Source: three-view drawing plus pictorial views. Frame: mm from the lowest corner of the part. A direction names the side the tool comes from. Give positions to 0.01 mm unless a question says otherwise; leave off trailing zeros. Write each loop counter-clockwise with the first axis right and the second up, starting at its lowest first coordinate (ties: lowest second). Pieces come first, ordered by that corner, then holes. Notation, with made-up numbers: (8.5, 50.5) -> (50.5, 50.5) arc R32 ccw to (50.5, 82.5) -> close; hole circle Ø5 at (46.5, 26). An arc over 180 degrees is marked (long way). Use a Markdown table: item, result. Add a question column.
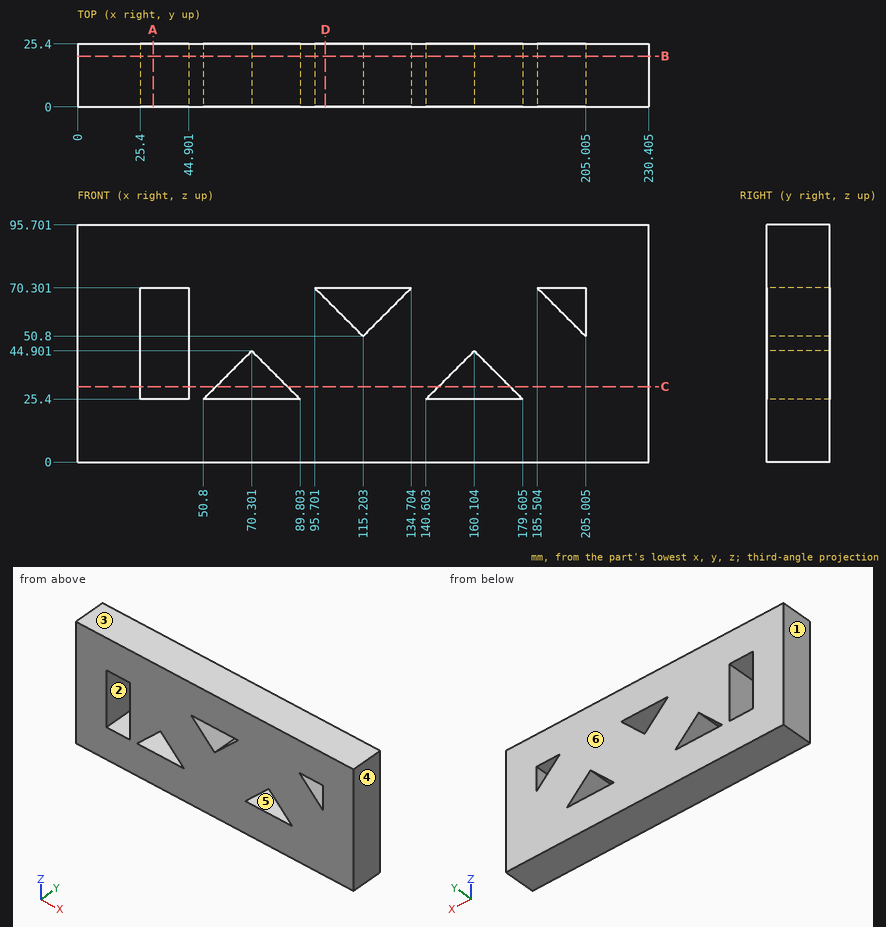
(1) Cut plane C-C on z = 30.5. Return the cut outline in (x, y) (1 decimal).
(2) Material intervals for L1, parallel to X at y = 7, z = 64 (1 decimal); L2, parallel to X at y = 20.5, z = 64.5 (1 decimal); L3, parallel to X at y = 24.25, z = 50.5 (1 decimal), sorted ascending.
(3) Cut plane B-B on y = 20.5. Return the cut outline in (x, z) (1 decimal).
(4) Cut plane A-A on x = 30.5. Return the cut outline in (y, z).
(5) Mould query, pull axis X, two halves, no side actions, for the marked faces 1, 2, 3 and 4. Classes: +X half, -X half, draft (parallel to the pull), parting line (faces both ways), or undercut.
(6) Cut plane D-D on x = 100. Return the cut outline in (y, z).
(7) First-contact query: pin 1 Ø7.5 at (y, z) = (18, 40.5) entering from -X; pin 2 Ø5 at (x, z) = (127, 67) entering from +Y. Flat tips, straight axial feed; report the tip coordinate or a pass-through.
(8) Access query for the marked faces 5 and 6. Directions: +Z, -Z, +X, -X, +Y, -Y. A direction counts if a zero-diameter tool reaches every point of the face in a straight line with its end or side. Return the directions, or none.
Output:
| question | item | result |
|---|---|---|
| 1 | outline | (0, 0) -> (25.4, 0) -> (25.4, 25.4) -> (0, 25.4) -> close; (44.9, 0) -> (55.9, 0) -> (55.9, 25.4) -> (44.9, 25.4) -> close; (84.7, 0) -> (145.7, 0) -> (145.7, 25.4) -> (84.7, 25.4) -> close; (174.5, 0) -> (230.4, 0) -> (230.4, 25.4) -> (174.5, 25.4) -> close |
| 2 | L1 | 0 to 25.4, 44.9 to 102, 128.4 to 191.8, 205 to 230.4 |
| 2 | L2 | 0 to 25.4, 44.9 to 101.5, 128.9 to 191.3, 205 to 230.4 |
| 2 | L3 | 0 to 25.4, 44.9 to 230.4 |
| 3 | outline | (0, 0) -> (230.4, 0) -> (230.4, 95.7) -> (0, 95.7) -> close; hole (25.4, 25.4) -> (44.9, 25.4) -> (44.9, 70.3) -> (25.4, 70.3) -> close; hole (50.8, 25.4) -> (89.8, 25.4) -> (70.3, 44.9) -> close; hole (95.7, 70.3) -> (115.2, 50.8) -> (134.7, 70.3) -> close; hole (140.6, 25.4) -> (179.6, 25.4) -> (160.1, 44.9) -> close; hole (185.5, 70.3) -> (205, 50.8) -> (205, 70.3) -> close |
| 4 | outline | (0, 0) -> (25.4, 0) -> (25.4, 25.4) -> (0, 25.4) -> close; (0, 70.3) -> (25.4, 70.3) -> (25.4, 95.7) -> (0, 95.7) -> close |
| 5 | face 1 | -X half |
| 5 | face 2 | undercut |
| 5 | face 3 | draft |
| 5 | face 4 | +X half |
| 6 | outline | (0, 0) -> (25.4, 0) -> (25.4, 66) -> (0, 66) -> close; (0, 70.3) -> (25.4, 70.3) -> (25.4, 95.7) -> (0, 95.7) -> close |
| 7 | pin 1 | x = 0 |
| 7 | pin 2 | through |
| 8 | face 5 | +Y, -Y |
| 8 | face 6 | +Z, -Z, +X, -X, +Y |
